Read the model definition and answer for the solid it produces. Units are mm, in the model's axes. A direction names the side the tool comes from. Round coordinates to 2 decimals unless told otherwise and drop trailing zeros. Write each loop counter-clockwise with the first axis right and the second up, starting at its lowest first coordinate (ties: lowest second). Pieces come first, ordered by that corner, then holes. Notation, with made-up numbers: M -17.5,64 L 22.5,64 A21 ccw 22.5,71 Z; hole C 24,-32 d5. An arc over 180 degrees is marked long. Use one line per item in the form item = value. Start each with the question number.
Autodesk Inventor part; units mm, degrees
ref_plane "YZ Plane" through (0, 0, 0) normal (1, 0, 0) x (0, 1, 0)
ref_plane "XZ Plane" through (0, 0, 0) normal (0, 1, 0) x (-1, 0, 0)
ref_plane "XY Plane" through (0, 0, 0) normal (0, 0, 1) x (1, 0, 0)
sketch "Sketch1" plane through (0, 0, 0) normal (0, 0, 1) x (1, 0, 0)
  line L0 (-9.525, 0) -> (9.525, 0)
  line L1 (9.525, 0) -> (9.525, 177.8)
  line L2 (9.525, 177.8) -> (-9.525, 177.8)
  line L3 (-9.525, 177.8) -> (-9.525, 0)
  point P0 (0, 0)
  point P1 (0, 0)
  dimension "d0" = 19.05
  dimension "d1" = 177.8
extrude "Extrusion1" add sketch "Sketch1" along normal blind 3.175
sketch "Sketch2" plane through (0, 0, 3.175) normal (0, 0, 1) x (1, 0, 0)
  arc A0 (-1.5, 11.8347) -> (1.5, 11.8347) centre (0, 9.525) ccw
  line L0 (-1.5, 11.8347) -> (1.5, 11.8347)
  line L1 (9.525, 0) -> (9.525, 177.8)
  line L2 (-9.525, 0) -> (9.525, 0)
  point P0 (0, 0)
  point P1 (0, 0)
  dimension "d4" = 2.754
  dimension "d5" = 3
  dimension "d8" = 9.525
  dimension "d9" = 9.525
extrude "Extrusion2" cut sketch "Sketch2" against normal blind 3.175
chamfer "Chamfer1" distance 3.175 angle 45 4 edges at (9.525, 0, 1.5875) (-9.525, 0, 1.5875) (9.525, 177.8, 1.5875) (-9.525, 177.8, 1.5875)
equation "\"d0\" = arm_distal_width"
equation "\"d1\" = arm_distal_length"
equation "\"d2\" = arm_distal_thickness"
equation "\"d10\" = arm_distal_thickness"
equation "\"base_width\" = 127"
equation "\"base_length\" = 177.8"
equation "\"base_height\" = 12.7"
equation "\"base_motor_standoff_length\" = 63.5"
equation "\"base_motor_standoff_height\" = 12.7"
equation "\"base_motor_standoff_thickness\" = 3.175"
equation "\"base_motor_standoff_offset\" = 0"
equation "\"waist_motor_cutout_diameter\" = 50.8"
equation "\"waist_cutout_overlap\" = 6.35"
equation "\"retention_poles_diameter\" = 6.35"
equation "\"turntable_bed_depth\" = 3.175"
equation "\"turntable_diameter\" = 101.6"
equation "\"turntable_spur_thickness\" = 6.35"
equation "\"turntable_thickness\" = 9.525"
equation "\"spine_diameter\" = 31.75"
equation "\"shoulder_height_offset\" = 25.4"
equation "\"shoulder_width\" = 69.85"
equation "\"shoulder_length\" = 50.8"
equation "\"shoulder_wall_thickness\" = 4.7625"
equation "\"arm_proximal_gear_diameter\" = 63.5"
equation "\"arm_proximal_gear_thickness\" = 9.525"
equation "\"shoulder_motor_gear_diameter\" = 25.4"
equation "\"arm_proximal_length\" = 228.6"
equation "\"arm_proximal_width\" = 12.7"
equation "\"arm_distal_length\" = 177.8"
equation "\"arm_distal_width\" = 19.05"
equation "\"arm_distal_thickness\" = 3.175"
equation "\"arm_proximal_thickness\" = 6.35"
equation "\"shoulder_motor_boss\" = 25.4"
equation "\"shoulder_gear_shaft_diameter\" = 12.7"
equation "\"shoulder_gear_thickness\" = 6.35"
equation "\"shoulder_gear_diameter\" = 63.5"
equation "\"spine_height\" = 25.4"
equation "\"turntable_retention_shaft_length\" = 152.4"
equation "\"turntable_height\" = 9.525"
equation "\"turntable_spur_width\" = 6.35"
equation "\"turntable_retention_shaft_diameter\" = 6.35"
equation "\"turntable_motor_support_width\" = 63.5"
equation "\"turntable_motor_boss\" = 25.4"
equation "\"turntable_motor_support_height\" = 25.4"
equation "\"turntable_motor_support_thickness\" = 3.175"
equation "\"base_cutout_diameter\" = 44.45"
equation "\"base_cutout_contact_angle\" = 70deg"
equation "\"arm_proximal_central_diameter\" = 25.4"
equation "\"arm_proximal_motor_boss\" = 25.4"
equation "\"turntable_ring_height\" = 9.525"
equation "\"turntable_ring_diameter\" = 19.05"
properties part number "arm_distal"
Q1. Find section B-B on x = -8. Write down the section's boundary in (y, z) (3 decimals), and give its area (3 significant figures).
Q2. A tool of negligible diameter and unlimited length cuts with its end or side. For faces 1 (the face through (0, 11.835, 2)), 2 (the face through (9.525, 88, 2)), from which of +Z, -Z, +X, -X, +Y, -Y can it reach the whole face along a straight path? Write none if from no direction.
Q3. Find section A-A on x = 0. Write down the section's boundary in (y, z) (3 decimals), and give its area (3 significant figures).
Q4. For a pull along Y with two mould halves and no side action, classify faces 3 (the face through (-7.92, 176.23, 1.57)), 4 (the face through (-0.099, 6.773, 1.61)), 5 (the face through (7.96, 1.61, 1.61)) as +Y half, -Y half, draft (parallel to the pull), parting line (faces both ways), or undercut.
Q5. Straight lines are drawn through the part: line 1 (Y direction, x = -1, z = 1.6); line 2 (Y direction, x = -0.5, z = 2.2); line 3 (Y direction, x = 7.25, z = 0.7). For each, find the intervals that lie inside material, in ascending order. Write a range as [from, to].
Response:
q1.outline = M 1.65,0 L 176.15,0 L 176.15,3.175 L 1.65,3.175 Z
q1.area = 554 mm²
q2.face_1 = +Z, -Z
q2.face_2 = +Z, -Z, +X, +Y, -Y
q3.outline = M 0,0 L 6.771,0 L 6.771,3.175 L 0,3.175 Z; M 11.835,0 L 177.8,0 L 177.8,3.175 L 11.835,3.175 Z
q3.area = 548 mm²
q4.face_3 = +Y half
q4.face_4 = undercut
q4.face_5 = -Y half
q5.line_1 = [0, 6.96], [11.83, 177.8]
q5.line_2 = [0, 6.82], [11.83, 177.8]
q5.line_3 = [0.9, 176.9]
